Study the drawing (mm; zero at the part's minimum x, y, z) and answer. Give positions to 0.01 mm unless a question says otherwise; leave off trailing zeros. Write each loop counter-clockwise with the first axis right and the second up, starting at its lowest first coordinate (ties: lowest second). Pieces come first, ordered by that corner, then holes. Notation, with made-up numbers: (33, -5) - (42, -5) arc R25 ccw to (42, 29) - close; hole circle Ø10 at (52, 6). An arc over 180 degrees is marked (long way). Return JSON: item names as keys, results as strings.
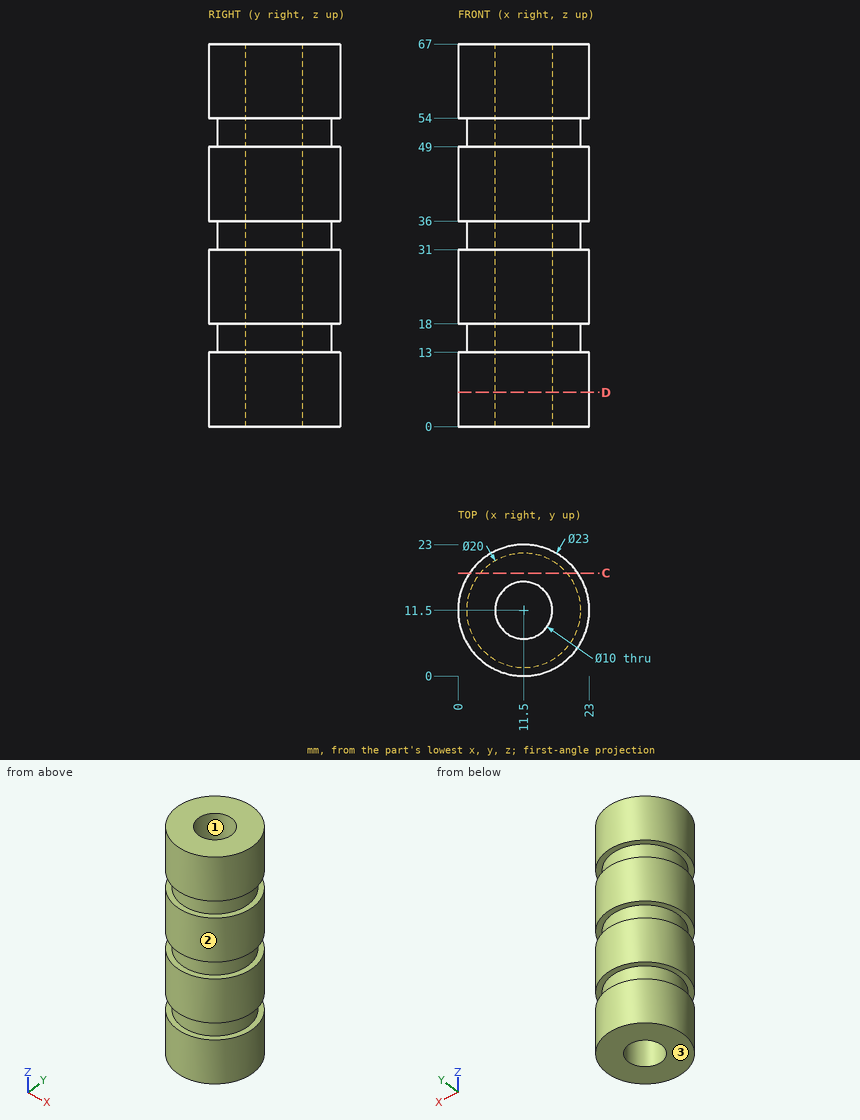
Item 1: The mould has two halves that part along Y. Classify the marked faces 1, 2 and 3: +Y half, -Y half, draft (parallel to the pull), parting line (faces both ways), or undercut.
Answer below:
{"face 1": "undercut", "face 2": "parting line", "face 3": "draft"}
Item 2: Consider L1, parallel to Z at x = 2.5, y = 16; L2, parallel to Y at x = 11.5, z = 30; L3, parallel to Y at x = 11.5, z = 35. Determine where each line is inside the solid, lowest interval first.
Answer below:
{"L1": "z = 0 to 13, 18 to 31, 36 to 49, 54 to 67", "L2": "y = 0 to 6.5, 16.5 to 23", "L3": "y = 1.5 to 6.5, 16.5 to 21.5"}
Item 3: Flat-ended cylindrical pins translate along their axes: P1, Ø2, axis at x = 14, z = 30, coming from the +Y side; P2, Ø6, axis at x = 19, z = 40.5, coming from the -Y side; P3, Ø6, axis at y = 17, z = 26, coming from the -X side (3 decimals). Find the tip coordinate at first contact, or state that the pin passes through.
Answer below:
{"P1": "stops at y = 22.9", "P2": "stops at y = 0.92", "P3": "stops at x = 0.275"}
Item 4: A cutting plane is placed at C-C on y = 18. Determine the outline of the cut face in (x, z), then the cut area to 3 significant figures.
Answer below:
{"outline": "(2.01, 0) - (20.99, 0) - (20.99, 13) - (19.1, 13) - (19.1, 18) - (20.99, 18) - (20.99, 31) - (19.1, 31) - (19.1, 36) - (20.99, 36) - (20.99, 49) - (19.1, 49) - (19.1, 54) - (20.99, 54) - (20.99, 67) - (2.01, 67) - (2.01, 54) - (3.9, 54) - (3.9, 49) - (2.01, 49) - (2.01, 36) - (3.9, 36) - (3.9, 31) - (2.01, 31) - (2.01, 18) - (3.9, 18) - (3.9, 13) - (2.01, 13) - close", "area": "1,210 mm²"}
Item 5: A cutting plane is placed at D-D on z = 6. Determine the outline of the cut face in (x, y).
Answer below:
{"outline": "circle Ø23 at (11.5, 11.5); hole circle Ø10 at (11.5, 11.5)"}
